Read the model definition and answer for the solid it produces. Units are mm, in the model's axes. Round coordinates to 2 decimals unless told otherwise and drop trailing zeros. Loops run counter-clockwise (first coordinate to the right, second up) from the corner with the lowest first, then second, coordinate; pieces in that order, holes last. Notation, with made-up numbers: (37.5, 56) -> (72.5, 56) arc R22 ccw to (72.5, 83) -> close; hole circle Ø10 at (21, -32). An arc over 180 degrees is marked (long way). Put each result on its own line as item: value.
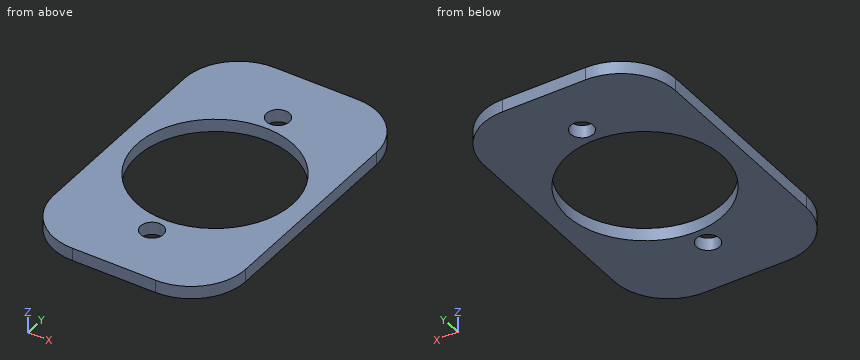
from build123d import *

# Parameters (mm, degrees)
BOSS_EXTRUDE1_DEPTH = 5
SKETCH4_W           = 53
SKETCH4_H           = 85
BOSS_EXTRUDE2_DEPTH = 3.5
SKETCH2_R           = 21.5
CUT_EXTRUDE1_DEPTH  = 74.391075752
SKETCH3_R           = 3.15
CUT_EXTRUDE2_DEPTH  = 74.391075752
SKETCH16_W          = 82.074163125
SKETCH16_H          = 140.053159095
SKETCH16_W_2        = 53
SKETCH16_H_2        = 85
LAZY_CUT_DEPTH      = 74.068461049
FILLET1_R           = 15
SKETCH17_W          = 53
SKETCH17_H          = 5
CUT_EXTRUDE7_DEPTH  = 90.175388981
SKETCH12_R          = 2.9
CUT_EXTRUDE3_DEPTH  = 3
SKETCH13_R          = 1.75
CUT_EXTRUDE4_DEPTH  = 51.386009963
CUT_EXTRUDE5_DEPTH  = 3
CUT_EXTRUDE6_DEPTH  = 1.5


with BuildPart() as part:
    # Sketch1 → Boss-Extrude1 (new body)
    with BuildSketch(Plane.XY):
        with BuildLine():
            Line((25, 65), (-25, 65))
            ThreePointArc((-25, 65), (-30.656854249, 62.656854249), (-33, 57))
            Line((-33, 57), (-33, -57))
            ThreePointArc((-33, -57), (-30.656854249, -62.656854249), (-25, -65))
            Line((-25, -65), (25, -65))
            ThreePointArc((25, -65), (30.656854249, -62.656854249), (33, -57))
            Line((33, -57), (33, 57))
            ThreePointArc((33, 57), (30.656854249, 62.656854249), (25, 65))
        make_face()
    extrude(amount=BOSS_EXTRUDE1_DEPTH)

    # Sketch4 → Boss-Extrude2 (add)
    with BuildSketch(Plane(origin=(0, 0, 0), x_dir=(-1, 0, 0), z_dir=(0, 0, -1))):
        Rectangle(SKETCH4_W, SKETCH4_H)
    extrude(amount=BOSS_EXTRUDE2_DEPTH)

    # Sketch2 → Cut-Extrude1 (cut, through all)
    with BuildSketch(Plane.XY.offset(5)):
        Circle(SKETCH2_R)
    extrude(amount=-CUT_EXTRUDE1_DEPTH, mode=Mode.SUBTRACT)

    # Sketch3 → Cut-Extrude2 (cut, through all)
    with BuildSketch(Plane.XY.offset(5)):
        with Locations((0, 26.5)):
            Circle(SKETCH3_R)
        with Locations((0, -26.5)):
            Circle(SKETCH3_R)
    extrude(amount=-CUT_EXTRUDE2_DEPTH, mode=Mode.SUBTRACT)

    # Sketch16 → lazy cut (cut, through all)
    with BuildSketch(Plane(origin=(0, 0, 0), x_dir=(-1, 0, 0), z_dir=(0, 0, -1))):
        with Locations((0.978866165, -0.150594795)):
            Rectangle(SKETCH16_W, SKETCH16_H)
        Rectangle(SKETCH16_W_2, SKETCH16_H_2, mode=Mode.SUBTRACT)
    extrude(amount=-LAZY_CUT_DEPTH, mode=Mode.SUBTRACT)

    # Fillet1
    fillet1_edges = [part.edges().sort_by_distance(p)[0] for p in [
        (-26.5, -42.5, 0.75),
        (-26.5, 42.5, 0.75),
        (26.5, 42.5, 0.75),
        (26.5, -42.5, 0.75),
    ]]
    fillet(fillet1_edges, radius=FILLET1_R)

    # Sketch17 → Cut-Extrude7 (cut, through all)
    with BuildSketch(Plane(origin=(0, 42.5, 0), x_dir=(1, 0, 0), z_dir=(0, 1, 0))):
        with Locations((0, -2.5)):
            Rectangle(SKETCH17_W, SKETCH17_H)
    extrude(amount=-CUT_EXTRUDE7_DEPTH, mode=Mode.SUBTRACT)

    # Sketch12 → Cut-Extrude3 (cut)
    with BuildSketch(Plane.XY.offset(5)):
        with Locations((-27.75, 59.75)):
            Circle(SKETCH12_R)
        with Locations((27.75, 59.75)):
            Circle(SKETCH12_R)
        with Locations((-27.75, -59.75)):
            Circle(SKETCH12_R)
        with Locations((27.75, -59.75)):
            Circle(SKETCH12_R)
    extrude(amount=-CUT_EXTRUDE3_DEPTH, mode=Mode.SUBTRACT)

    # Sketch13 → Cut-Extrude4 (cut, through all)
    with BuildSketch(Plane.XY.offset(2)):
        with Locations((-27.75, 59.75)):
            Circle(SKETCH13_R)
        with Locations((27.75, 59.75)):
            Circle(SKETCH13_R)
        with Locations((27.75, -59.75)):
            Circle(SKETCH13_R)
        with Locations((-27.75, -59.75)):
            Circle(SKETCH13_R)
    extrude(amount=-CUT_EXTRUDE4_DEPTH, mode=Mode.SUBTRACT)

    # Sketch14 → Cut-Extrude5 (cut)
    with BuildSketch(Plane.XY.offset(5)):
        with BuildLine():
            Line((-5.5, 26.5), (-5.5, -26.5))
            ThreePointArc((-5.5, -26.5), (0, -32), (5.5, -26.5))
            Line((5.5, -26.5), (5.5, 26.5))
            ThreePointArc((5.5, 26.5), (0, 32), (-5.5, 26.5))
        make_face()
    extrude(amount=-CUT_EXTRUDE5_DEPTH, mode=Mode.SUBTRACT)

    # Sketch15 → Cut-Extrude6 (cut)
    with BuildSketch(Plane.XY.offset(5)):
        with BuildLine():
            Line((-2.5, 65), (-2.5, 31.398979486))
            ThreePointArc((-2.5, 31.398979486), (0, 32), (2.5, 31.398979486))
            Line((2.5, 31.398979486), (2.5, 65))
            Line((2.5, 65), (-2.5, 65))
        make_face()
        with BuildLine():
            Line((-27.75, 13.75), (-20.879116361, 13.75))
            ThreePointArc((-20.879116361, 13.75), (-14.747047157, 20.187238547), (-6.75, 24.071508054))
            Line((-6.75, 24.071508054), (-6.75, 59.75))
            Line((-6.75, 59.75), (-21.75, 59.75))
            ThreePointArc((-21.75, 59.75), (-23.507359313, 55.507359313), (-27.75, 53.75))
            Line((-27.75, 53.75), (-27.75, 13.75))
        make_face()
        with BuildLine():
            Line((27.75, 13.75), (20.879116361, 13.75))
            ThreePointArc((20.879116361, 13.75), (14.747047157, 20.187238547), (6.75, 24.071508054))
            Line((6.75, 24.071508054), (6.75, 59.75))
            Line((6.75, 59.75), (21.75, 59.75))
            ThreePointArc((21.75, 59.75), (23.507359313, 55.507359313), (27.75, 53.75))
            Line((27.75, 53.75), (27.75, 13.75))
        make_face()
        with BuildLine():
            Line((27.75, -53.75), (27.75, -13.75))
            Line((27.75, -13.75), (20.879116361, -13.75))
            ThreePointArc((20.879116361, -13.75), (14.747047157, -20.187238547), (6.75, -24.071508054))
            Line((6.75, -24.071508054), (6.75, -59.75))
            Line((6.75, -59.75), (21.75, -59.75))
            ThreePointArc((21.75, -59.75), (23.507359313, -55.507359313), (27.75, -53.75))
        make_face()
        with BuildLine():
            Line((2.5, -65), (2.5, -31.398979486))
            ThreePointArc((2.5, -31.398979486), (0, -32), (-2.5, -31.398979486))
            Line((-2.5, -31.398979486), (-2.5, -65))
            Line((-2.5, -65), (2.5, -65))
        make_face()
        with BuildLine():
            Line((-6.75, -59.75), (-6.75, -24.071508054))
            ThreePointArc((-6.75, -24.071508054), (-14.747047157, -20.187238547), (-20.879116361, -13.75))
            Line((-20.879116361, -13.75), (-27.75, -13.75))
            Line((-27.75, -13.75), (-27.75, -53.75))
            ThreePointArc((-27.75, -53.75), (-23.507359313, -55.507359313), (-21.75, -59.75))
            Line((-21.75, -59.75), (-6.75, -59.75))
        make_face()
    extrude(amount=-CUT_EXTRUDE6_DEPTH, mode=Mode.SUBTRACT)


solid = part.part
Item 1: Find the intervals of material crossed by line 1 along Y through (x, z) = (0, -0.9); line 2 along Y through (x, z) = (-19, -2.2); line 3 along Y through (x, z) = (-5.5, -1.6), in increasing order.
Derived:
line 1: y = -42.5 to -29.65, -23.35 to -21.5, 21.5 to 23.35, 29.65 to 42.5
line 2: y = -40.49 to -10.06, 10.06 to 40.49
line 3: y = -42.5 to -20.78, 20.78 to 42.5
Item 2: The part is cut by section C-C (z = -1.8). Determine the outline of the cut face in (x, y).
Derived:
outline: (-26.5, -27.5) arc R15 ccw to (-11.5, -42.5) -> (11.5, -42.5) arc R15 ccw to (26.5, -27.5) -> (26.5, 27.5) arc R15 ccw to (11.5, 42.5) -> (-11.5, 42.5) arc R15 ccw to (-26.5, 27.5) -> close; hole circle Ø43 at (0, 0); hole circle Ø6.3 at (0, -26.5); hole circle Ø6.3 at (0, 26.5)
Item 3: The part is cut by section B-B (x = 0). Determine the outline of the cut face in (y, z), then the cut area to 3 significant figures.
Derived:
outline: (-42.5, -3.5) -> (-29.65, -3.5) -> (-29.65, 0) -> (-42.5, 0) -> close; (-23.35, -3.5) -> (-21.5, -3.5) -> (-21.5, 0) -> (-23.35, 0) -> close; (21.5, -3.5) -> (23.35, -3.5) -> (23.35, 0) -> (21.5, 0) -> close; (29.65, -3.5) -> (42.5, -3.5) -> (42.5, 0) -> (29.65, 0) -> close
area: 103 mm^2
Item 4: The part is cut by section D-D (x = -20). Determine the outline of the cut face in (y, z), then the cut area to 3 significant figures.
Derived:
outline: (-39.86, -3.5) -> (-7.89, -3.5) -> (-7.89, 0) -> (-39.86, 0) -> close; (7.89, -3.5) -> (39.86, -3.5) -> (39.86, 0) -> (7.89, 0) -> close
area: 224 mm^2
Item 5: A flat-ended cylindrical pin translates along its axis: pin 1 Ø5 at (x, y) = (0, 26.5) entering from +Z (3 decimals). Find the tip coordinate at first contact, or state that the pin passes through.
Derived:
pin 1: passes through
Item 6: The part is cut by section A-A (y = -26.5). Determine the outline of the cut face in (x, z), then the cut area to 3 significant figures.
Derived:
outline: (-26.5, -3.5) -> (-3.15, -3.5) -> (-3.15, 0) -> (-26.5, 0) -> close; (3.15, -3.5) -> (26.5, -3.5) -> (26.5, 0) -> (3.15, 0) -> close
area: 163 mm^2
